Can you work these out from the model? Positions are in its coordinate system, mm. Face numbers are marked on the shaded views. A direction names the side the tool comes from. Round coordinates to 2 decimals unless told otherwise and drop trailing zeros. Order: outer loops, then holes, each group sorted by start corner. A loop starts at its lowest first (then second) coordinate and runs counter-clockwise, first axis right, second up. Notation, with made-up numbers: (27, 22) -> (57, 22) arc R32 cw to (57, 59) -> close; hole circle Ø1 at (82, 5). An arc over 180 degrees is marked (long way). One line per item, written item: value.
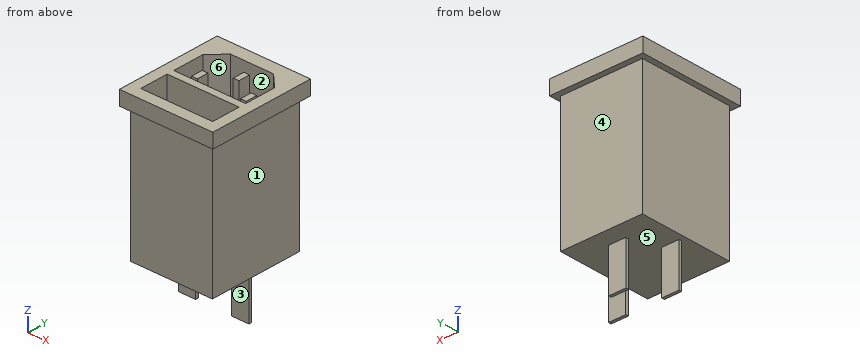
```python
from build123d import *

# Parameters (mm, degrees)
SKETCH1_W           = 28.5
SKETCH1_H           = 33
BOSS_EXTRUDE1_DEPTH = 46
SKETCH2_W           = 32.5
SKETCH2_H           = 37
BOSS_EXTRUDE2_DEPTH = 5
SKETCH3_W           = 25
SKETCH3_H           = 10
CUT_EXTRUDE1_DEPTH  = 17
SKETCH4_W           = 2
SKETCH4_H           = 4
BOSS_EXTRUDE3_DEPTH = 15
SKETCH5_W           = 6
SKETCH5_H           = 1
BOSS_EXTRUDE4_DEPTH = 15


with BuildPart() as part:
    # Sketch1 → Boss-Extrude1 (new body)
    with BuildSketch(Plane.XY):
        Rectangle(SKETCH1_W, SKETCH1_H)
    extrude(amount=BOSS_EXTRUDE1_DEPTH)

    # Sketch2 → Boss-Extrude2 (add)
    with BuildSketch(Plane.XY.offset(46)):
        Rectangle(SKETCH2_W, SKETCH2_H)
    extrude(amount=BOSS_EXTRUDE2_DEPTH)

    # Sketch3 → Cut-Extrude1 (cut)
    with BuildSketch(Plane.XY.offset(51)):
        Polygon((12.5, -2), (-12.5, -2), (-12.5, 9), (-7.5, 14), (7.5, 14), (12.5, 9), align=None)
        with Locations((0, -9.5)):
            Rectangle(SKETCH3_W, SKETCH3_H)
    extrude(amount=-CUT_EXTRUDE1_DEPTH, mode=Mode.SUBTRACT)

    # Sketch4 → Boss-Extrude3 (add)
    with BuildSketch(Plane.XY.offset(34)):
        with Locations((-8.5, 3.5)):
            Rectangle(SKETCH4_W, SKETCH4_H)
        with Locations((0, 10)):
            Rectangle(SKETCH4_W, SKETCH4_H)
        with Locations((8.5, 3.5)):
            Rectangle(SKETCH4_W, SKETCH4_H)
    extrude(amount=BOSS_EXTRUDE3_DEPTH)

    # Sketch5 → Boss-Extrude4 (add)
    with BuildSketch(Plane(origin=(0, 0, 0), x_dir=(-1, 0, 0), z_dir=(0, 0, -1))):
        with Locations((-9.25, 0)):
            Rectangle(SKETCH5_W, SKETCH5_H)
        with Locations((0, 10)):
            Rectangle(SKETCH5_W, SKETCH5_H)
        with Locations((9.25, 0)):
            Rectangle(SKETCH5_W, SKETCH5_H)
    extrude(amount=BOSS_EXTRUDE4_DEPTH)


solid = part.part
```
Q1. On a 3-axis mill with a long thin cutter (end or side, diameter ignored), from which of +Z, -Z, +X, -X, +Y, -Y can I reach the whole of each face in a straight line? I mean the marked faces 1, 2 and 3. Say none if no direction works.
Answers below:
face 1: -Z, +X, +Y, -Y
face 2: +Z
face 3: -Z, +X, -X, -Y
Q2. I want a section at A-A on z = -8.5. List the corners of the cut face in (x, y) for me, plus the area to 3 significant figures.
Answers below:
outline: (-12.25, -0.5) -> (-6.25, -0.5) -> (-6.25, 0.5) -> (-12.25, 0.5) -> close; (-3, 9.5) -> (3, 9.5) -> (3, 10.5) -> (-3, 10.5) -> close; (6.25, -0.5) -> (12.25, -0.5) -> (12.25, 0.5) -> (6.25, 0.5) -> close
area: 18.0 mm^2
Q3. Will these pins go through, and if not, where does the flat tip stop? pin 1 Ø4 at (y, z) = (-14, 4.5) entering from +X; pin 2 Ø1.6 at (x, y) = (8.5, 4) entering from +Z; pin 3 Ø5 at (x, z) = (-9.5, -10.5) entering from +Y.
Answers below:
pin 1: x = 14.25
pin 2: z = 49
pin 3: y = 0.5
Q4. I want a section at B-B on z = 36. List the corners of the cut face in (x, y) for me, plus the area to 4 significant figures.
Answers below:
outline: (-14.25, -16.5) -> (14.25, -16.5) -> (14.25, 16.5) -> (-14.25, 16.5) -> close; (-9.5, 1.5) -> (-7.5, 1.5) -> (-7.5, 5.5) -> (-9.5, 5.5) -> close; (-1, 8) -> (1, 8) -> (1, 12) -> (-1, 12) -> close; (7.5, 1.5) -> (9.5, 1.5) -> (9.5, 5.5) -> (7.5, 5.5) -> close; hole (-12.5, -14.5) -> (12.5, -14.5) -> (12.5, -4.5) -> (-12.5, -4.5) -> close; hole (-12.5, -2) -> (12.5, -2) -> (12.5, 9) -> (7.5, 14) -> (-7.5, 14) -> (-12.5, 9) -> close
area: 339.5 mm^2
Q5. Please list where these lines run through material, in increasing order: line 1 along Y through (x, z) = (6, 37.5); line 2 along X through (y, z) = (-1, 45); line 3 along Y through (x, z) = (10, 39).
Answers below:
line 1: -16.5 to -14.5, -4.5 to -2, 14 to 16.5
line 2: -14.25 to -12.5, 12.5 to 14.25
line 3: -16.5 to -14.5, -4.5 to -2, 11.5 to 16.5
Q6. I want a section at D-D on y = 15. List the corners of the cut face in (x, z) for me.
Answers below:
outline: (-16.25, 46) -> (-14.25, 46) -> (-14.25, 0) -> (14.25, 0) -> (14.25, 46) -> (16.25, 46) -> (16.25, 51) -> (-16.25, 51) -> close
Q7. I want a section at C-C on x = -8.5. List the corners of the cut face in (y, z) for me.
Answers below:
outline: (-18.5, 46) -> (-16.5, 46) -> (-16.5, 0) -> (-0.5, 0) -> (-0.5, -15) -> (0.5, -15) -> (0.5, 0) -> (16.5, 0) -> (16.5, 46) -> (18.5, 46) -> (18.5, 51) -> (13, 51) -> (13, 34) -> (5.5, 34) -> (5.5, 49) -> (1.5, 49) -> (1.5, 34) -> (-2, 34) -> (-2, 51) -> (-4.5, 51) -> (-4.5, 34) -> (-14.5, 34) -> (-14.5, 51) -> (-18.5, 51) -> close
Q8. We'd pull the mould along Y, two halves only. Please class the marked faces 4, 5 and 6: released by +Y, released by -Y, zero draft, split by the parting line, or undercut.
Answers below:
face 4: released by +Y
face 5: zero draft
face 6: undercut
